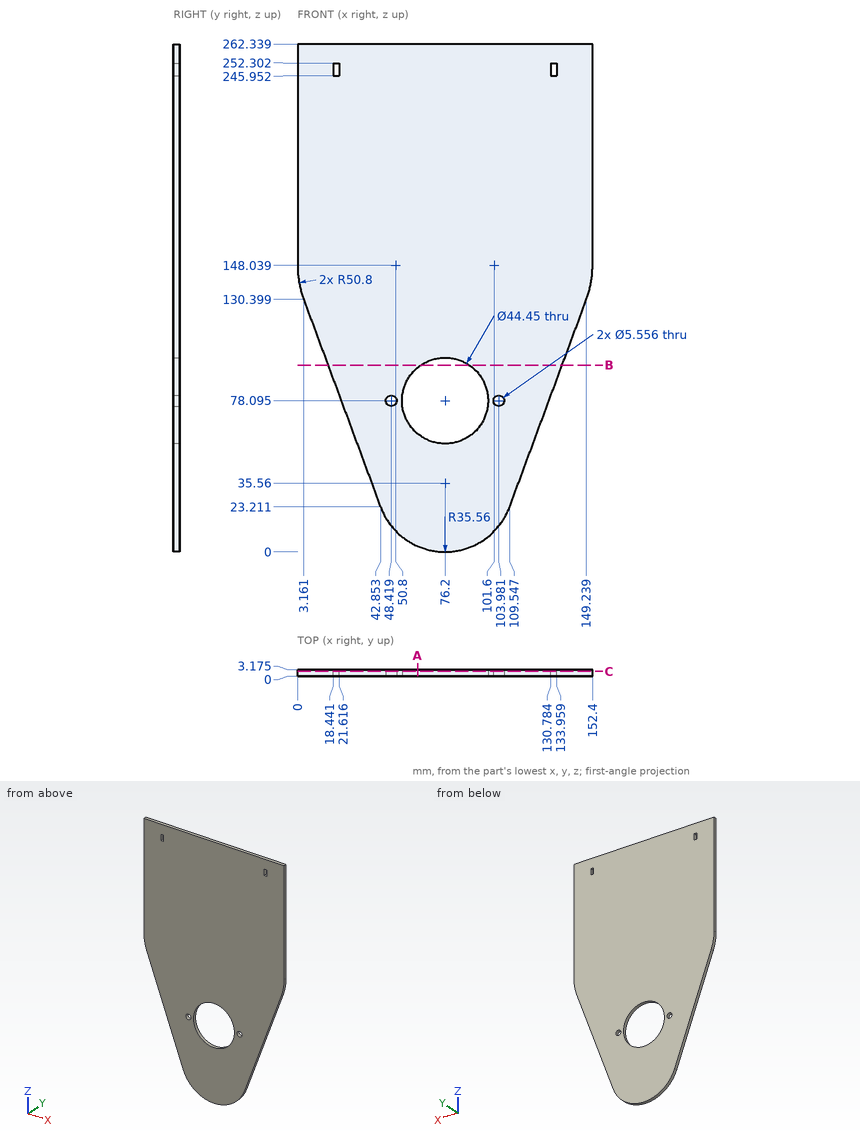
Geometry check sheet. Reference: drawing and pictorial views, mm from the part's lowest x, y, z. Coordinates: 2 decimals unless noted, no trailing zeros. Order: outer loops, then holes, each group sorted by start corner. A loop starts at its lowest first (then second) coordinate and runs counter-clockwise, first axis right, second up. Notation, with made-up numbers: (-7, 56) - (2, 56) arc R20 ccw to (2, 61) - close; hole circle Ø7 at (-10.5, 81). An arc over 180 degrees is marked (long way). One line per item, written item: value.
(1) Sectioned sample at C-C (y = 2.35). Count the separate pieces of the cut face and the enclosed holes in it, and give its area (3 significant figures).
Data:
separate pieces: 1
enclosed holes: 5
area: 31,000 mm^2
(2) Thickness scan on probe 1 along Z at (x, y) = (103.5, 0.7) (1 decimal); probe 2 along X at (y, z) = (1.9, 88) (1 decimal); probe 3 along Z at (x, y) = (105, 1) (1 decimal). Record the ranges inside material, lowest first. Write a range as from..to.
Data:
probe 1: z = 12.8..75.4, 80.8..262.3
probe 2: x = 18.9..56.3, 96.1..133.5
probe 3: z = 14.7..75.5, 80.7..262.3
(3) Sectioned sample at B-B (z = 96.5). Enter the section's corners in (x, y) (1 decimal), and give its area (3 significant figures).
Data:
outline: (15.7, 0) - (63.7, 0) - (63.7, 3.2) - (15.7, 3.2) - close; (88.7, 0) - (136.7, 0) - (136.7, 3.2) - (88.7, 3.2) - close
area: 305 mm^2
(4) Sectioned sample at A-A (x = 62). Enter the section's corners in (y, z) (1 decimal), and give its area (3 significant figures).
Data:
outline: (0, 3) - (3.2, 3) - (3.2, 61) - (0, 61) - close; (0, 95.2) - (3.2, 95.2) - (3.2, 262.3) - (0, 262.3) - close
area: 715 mm^2
(5) Depth check by flat-ended pin: pin 1 Ø3.5 at (x, z) = (103.98, 78.1) entering from -Y. Enter the tip coordinate at first touch or a pass-through.
Data:
pin 1: passes through
